Input: dimensioned drawing with shaded views. Units: mm. Origin: part minimum x, y, z. A direction names the side the tool comes from. Round coordinates to 2 decimals unless told otherwise and drop trailing zeros. Write each loop counter-clockwise with the first axis right and the second up, starting at its lowest first coordinate (ties: lowest second). Pieces come first, ordered by that corner, then holes. Notation, with made-up numbers: (-34, 85) - (-13, 85) arc R19 cw to (-13, 105) - close; hole circle Ø11 at (61, 21). An arc over 180 degrees is marked (long way). Use one line per item in the form item = value.
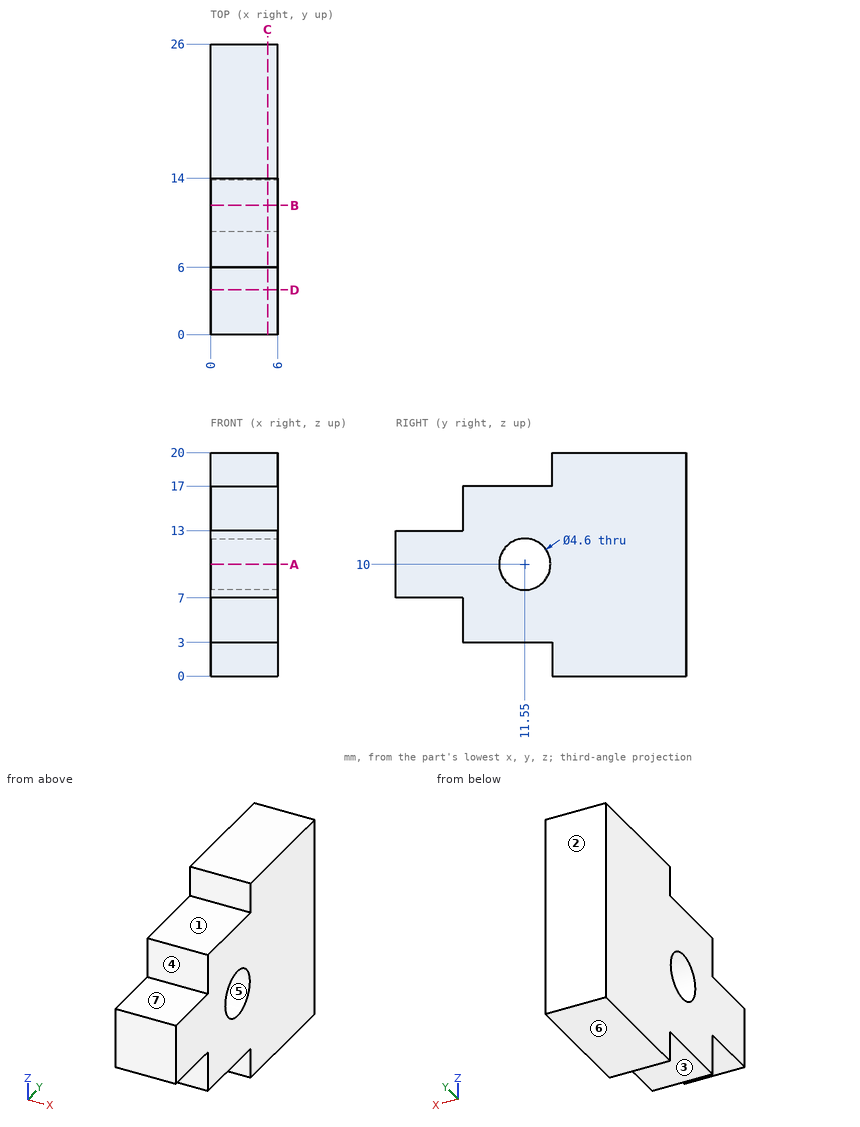
(1) Cut plane D-D on y = 4. Output: boundary loops of the cut face in (x, z), then the cut area to 3 significant figures.
Derived:
outline = (0, 7) - (6, 7) - (6, 13) - (0, 13) - close
area = 36.0 mm^2
(2) First-contact query: pin 1 Ø1.2 at (x, z) = (1.5, 15.5) entering from -Y; pin 2 Ø1.5 at (y, z) = (19, 14) entering from -X; pin 3 Ø1.8 at (x, y) = (3, 1.5) entering from -Z; pin 4 Ø2 at (x, y) = (2.5, 9) entering from +Z. Flat tips, straight axial feed; report the tip coordinate or a pass-through.
Derived:
pin_1 = 6
pin_2 = 0
pin_3 = 7
pin_4 = 17
(3) Material intervals for L1, parallel to Y at x = 3.1, z = 10; L2, parallel to Y at x = 4.1, z = 4; L3, parallel to Y at x = 0.4, z = 2, sorted ascending.
Derived:
L1 = 0 to 9.25, 13.85 to 26
L2 = 6 to 26
L3 = 14 to 26
(4) Access query for the marked faces 1, 2 and 3. Directions: +Z, -Z, +X, -X, +Y, -Y. A direction counts if a zero-diameter tool reaches every point of the face in a straight line with its end or side. Return the directions, or none.
Derived:
face_1 = +Z, +X, -X, -Y
face_2 = +Z, -Z, +X, -X, +Y
face_3 = -Z, +X, -X, -Y
(5) Cut plane B-B on y = 11.55. Output: boundary loops of the cut face in (x, z), then the cut area to 3 significant figures.
Derived:
outline = (0, 3) - (6, 3) - (6, 7.7) - (0, 7.7) - close; (0, 12.3) - (6, 12.3) - (6, 17) - (0, 17) - close
area = 56.4 mm^2
(6) Cut plane C-C on x = 5.1. Output: boundary loops of the cut face in (y, z).
Derived:
outline = (0, 7) - (6, 7) - (6, 3) - (14, 3) - (14, 0) - (26, 0) - (26, 20) - (14, 20) - (14, 17) - (6, 17) - (6, 13) - (0, 13) - close; hole circle Ø4.6 at (11.55, 10)
(7) Draft query along Z for the marked faces 4, 5, 6 and 7. Return one class per face: released by +Z, released by -Z, zero draft, split by the parting line, or undercut.
Derived:
face_4 = zero draft
face_5 = undercut
face_6 = released by -Z
face_7 = released by +Z
(8) Cut plane A-A on z = 10. Output: boundary loops of the cut face in (x, y), then the cut area to 3 significant figures.
Derived:
outline = (0, 0) - (6, 0) - (6, 9.25) - (0, 9.25) - close; (0, 13.85) - (6, 13.85) - (6, 26) - (0, 26) - close
area = 128 mm^2
